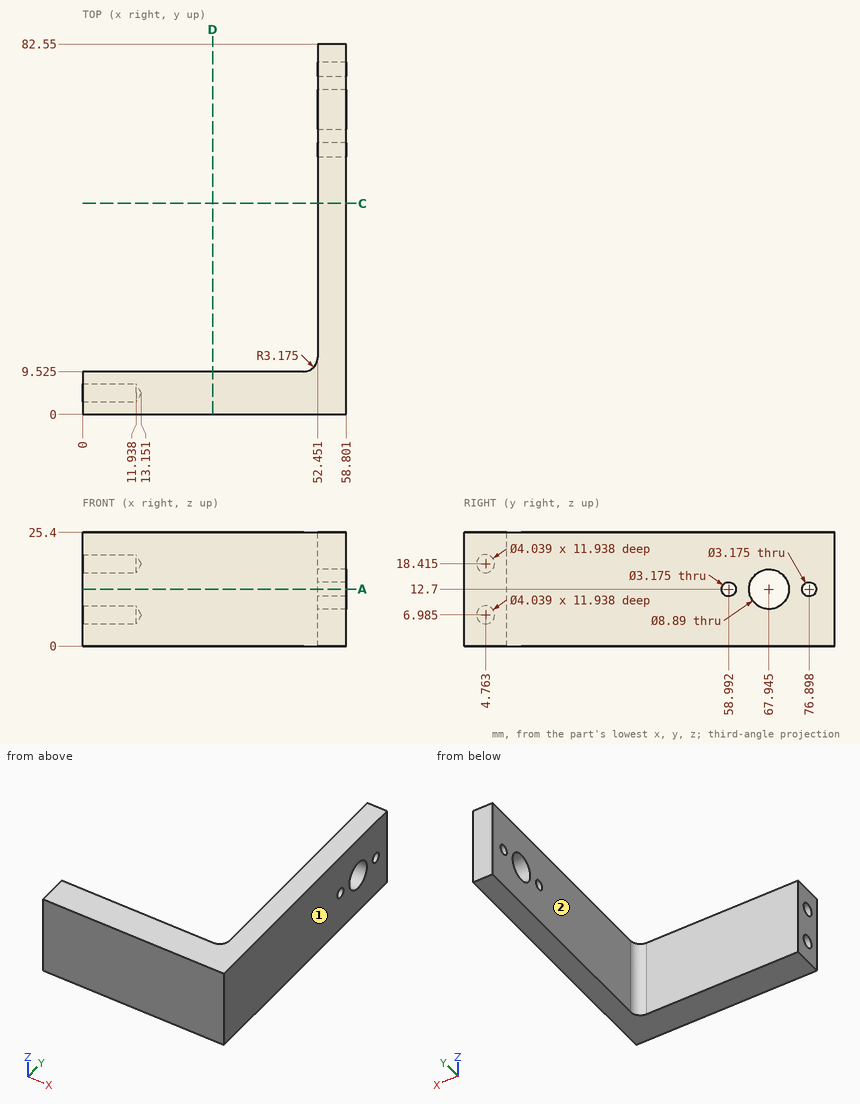
Source: three-view drawing plus pictorial views. Frame: mm from the lowest corner of the part. A direction names the side the tool comes from. Give positions to 0.01 mm unless a question says otherwise; leave off trailing zeros. Order: outer loops, then holes, each group sorted by start corner. A loop starts at its lowest first (then second) coordinate and runs counter-clockwise, first axis right, second up. Notation, with made-up numbers: M 35,-38 L 69,-38 A20 ccw 69,-34 Z; hole C 68,18.5 d6. An arc over 180 degrees is marked long. Return JSON: item names as keys, results as strings.
Item 1: Cut plane D-D (x = 29). Return loops of the section in (y, z) (1 decimal).
Solutions:
{"outline": "M 0,0 L 9.5,0 L 9.5,25.4 L 0,25.4 Z"}
Item 2: Cut plane C-C (y = 47). Return loops of the section in (x, z), then the cut area to 3 significant figures.
Solutions:
{"outline": "M 52.45,0 L 58.8,0 L 58.8,25.4 L 52.45,25.4 Z", "area": "161 mm^2"}
Item 3: Access query for the marked faces 1 and 2. Directions: +Z, -Z, +X, -X, +Y, -Y. A direction counts if a zero-diameter tool reaches every point of the face in a straight line with its end or side. Return the directions, or none.
Solutions:
{"face 1": "+Z, -Z, +X, +Y, -Y", "face 2": "+Z, -Z, -X, +Y"}
Item 4: Ray query, probe 1 along X at (y, z) = (47.5, 14.25); probe 2 along Y at (x, z) = (23, 13) (1 decimal); probe 3 along Z at (x, y) = (56, 71). Return the intervals inside material, ascending.
Solutions:
{"probe 1": "52.45 to 58.8", "probe 2": "0 to 9.5", "probe 3": "0 to 9.47, 15.93 to 25.4"}
Item 5: Cut plane A-A (z = 12.7). State how many separate pieces and enclosed holes the cut face has, then the cut area to 3 significant figures.
Solutions:
{"separate pieces": "4", "enclosed holes": "0", "area": "929 mm^2"}
Item 6: First-contact query: P1, Ø4, axis at x = 41.5, z = 3.5, coming from the +Y side (1 decimal); P2, Ø1, axis at y = 58.5, z = 6, coming from the -X side. Flat tips, straight axial feed; report the tip coordinate or a pass-through.
Solutions:
{"P1": "y = 9.5", "P2": "x = 52.45"}
